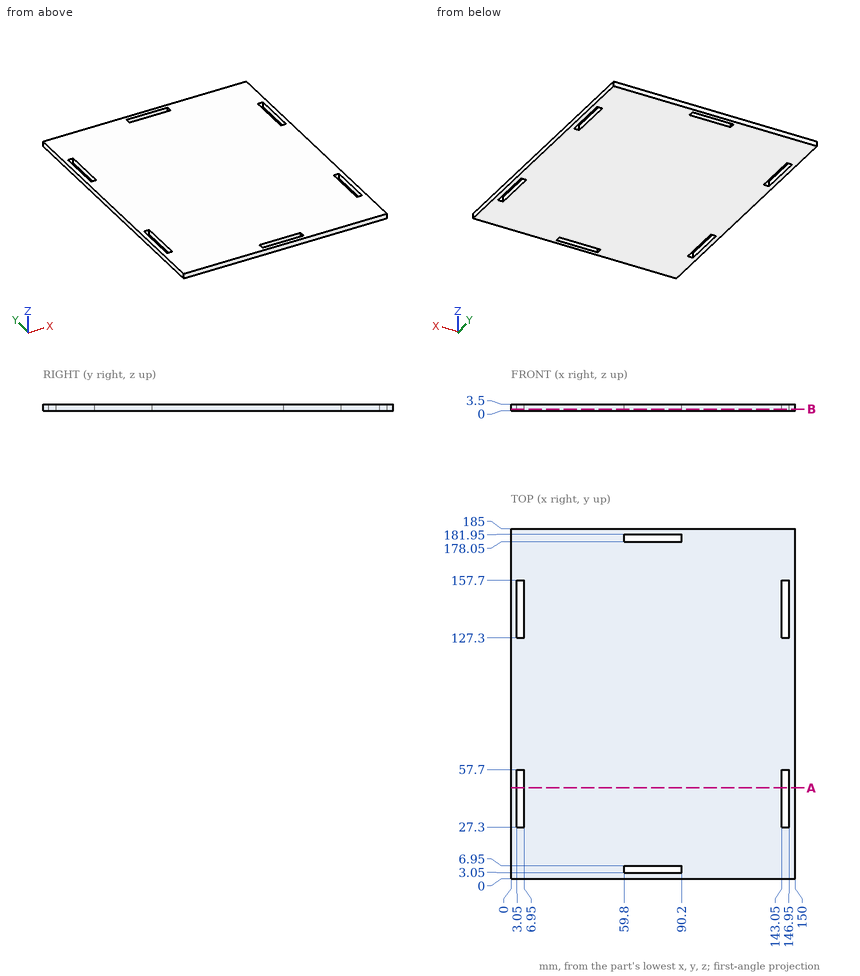
Can you work these out from the drawing? Everything is in mm from the part's minimum corner. Coordinates: 2 decimals unless noted, no trailing zeros. Loops run counter-clockwise (first coordinate to the right, second up) from the corner with the lowest first, then second, coordinate; pieces in that order, holes last.
1) I need wall thicknesses on probe 1 along Y at (x, z) = (81, 3.05); probe 2 along X at (y, z) = (146, 1.8). Which ranges of each line are inside material? Lowest first, please.
2) For pin 1 (1.8 mm diameter, centred on x = 5, z = 1, fed in from -Y), with a flat end and sliding along its axis, tell me the tip position at first contact or that it passes through.
3) Imagine slicing it at A-A on y = 48. List the corners of the cut face in (x, z) for me.
4) Imagine slicing it at B-B on z = 0.8. List the corners of the cut face in (x, y) for me, plus the area to 3 significant figures.
Completed:
1. probe 1: y = 0 to 3.05, 6.95 to 178.05, 181.95 to 185
1. probe 2: x = 0 to 3.05, 6.95 to 143.05, 146.95 to 150
2. pin 1: stops at y = 0
3. outline: (0, 0) - (3.05, 0) - (3.05, 3.5) - (0, 3.5) - close; (6.95, 0) - (143.05, 0) - (143.05, 3.5) - (6.95, 3.5) - close; (146.95, 0) - (150, 0) - (150, 3.5) - (146.95, 3.5) - close
4. outline: (0, 0) - (150, 0) - (150, 185) - (0, 185) - close; hole (3.05, 27.3) - (6.95, 27.3) - (6.95, 57.7) - (3.05, 57.7) - close; hole (3.05, 127.3) - (6.95, 127.3) - (6.95, 157.7) - (3.05, 157.7) - close; hole (59.8, 3.05) - (90.2, 3.05) - (90.2, 6.95) - (59.8, 6.95) - close; hole (59.8, 178.05) - (90.2, 178.05) - (90.2, 181.95) - (59.8, 181.95) - close; hole (143.05, 27.3) - (146.95, 27.3) - (146.95, 57.7) - (143.05, 57.7) - close; hole (143.05, 127.3) - (146.95, 127.3) - (146.95, 157.7) - (143.05, 157.7) - close
4. area: 27,000 mm2
